Part model, mm, in its own coordinate system. Round coordinates to 2 decimals unless told otherwise and drop trailing zeros. Write each loop counter-clockwise with the first axis right and the second up, starting at its lowest first coordinate (ties: lowest second). Pieces come first, ordered by that corner, then holes. Notation, with made-up numbers: M 32,33 L 37,33 A19 cw 37,49 Z; hole C 11,37.5 d8. An arc over 180 degrees is marked long. Use a Markdown table: item, result. Add a question column.
1) Slice it at D-D on z = 4.75. Write the cut outline in (x, y) (1 decimal).
2) Slice it at C-C on z = 3.25. Write the cut outline in (x, y), plus the area to 3 significant figures.
3) Wall check: probe 1 along Y at (x, z) = (0, 1.5); probe 2 along Y at (x, z) = (0, 4.5); probe 3 along Y at (x, z) = (-7, 1.75). Give the ranges that are in metal, low to high.
4) Drop a flat-ended pin along its axis: P1, Ø1, axis at x = 5.5, z = 3, coming from the +Y side. Give the stop position or say it passes through.
5) Two-plate mould, pull along X, no slides. Class faces 1 (the face through (-2.17, -9.76, 1.97)), 2 (the face through (0, -2, 7)), 3 (the face through (6.2, -0.6, 3.5)): released by +X, released by -X, zero draft, split by the parting line, or undercut.
6) Slice it at A-A on y = 0. Write the cut outline in (x, z), plus the area to 4 significant figures.
```python
from build123d import *

# Parameters (mm, degrees)
SKETCH1_R           = 10
SKETCH1_R_2         = 1.6
BOSS_EXTRUDE1_DEPTH = 7
SKETCH2_R           = 1
CUT_EXTRUDE1_DEPTH  = 7
CHAMFER2_SIZE       = 3
CHAMFER2_SIZE2      = 1.25


with BuildPart() as part:
    # Sketch1 → Boss-Extrude1 (new body)
    with BuildSketch(Plane.XY):
        Circle(SKETCH1_R)
        Circle(SKETCH1_R_2, mode=Mode.SUBTRACT)
    extrude(amount=BOSS_EXTRUDE1_DEPTH)

    # Sketch2 → Cut-Extrude1 (cut)
    with BuildSketch(Plane.XY.offset(7)):
        with Locations((7, 0)):
            Circle(SKETCH2_R)
        with Locations((0, -7)):
            Circle(SKETCH2_R)
        with Locations((-7, 0)):
            Circle(SKETCH2_R)
        with Locations((0, 7)):
            Circle(SKETCH2_R)
    extrude(amount=-CUT_EXTRUDE1_DEPTH, mode=Mode.SUBTRACT)

    # Chamfer2
    chamfer2_edges = [part.edges().sort_by_distance(p)[0] for p in [
        (-10, 0, 7),
    ]]
    chamfer2_side = [part.faces().sort_by_distance(p)[0] for p in [
        (-10, 0, 3.5),
    ]]
    chamfer(chamfer2_edges, length=CHAMFER2_SIZE, length2=CHAMFER2_SIZE2, reference=chamfer2_side[0])


solid = part.part
```
Entries:
| question | item | result |
|---|---|---|
| 1 | outline | C 0,0 d19.4; hole C -7,0 d2; hole C 0,0 d3.2; hole C 0,-7 d2; hole C 0,7 d2; hole C 7,0 d2 |
| 2 | outline | C 0,0 d20; hole C -7,0 d2; hole C 0,0 d3.2; hole C 0,-7 d2; hole C 0,7 d2; hole C 7,0 d2 |
| 2 | area | 294 mm^2 |
| 3 | probe 1 | y = -10 to -8, -6 to -1.6, 1.6 to 6, 8 to 10 |
| 3 | probe 2 | y = -9.79 to -8, -6 to -1.6, 1.6 to 6, 8 to 9.79 |
| 3 | probe 3 | y = -7.14 to -1, 1 to 7.14 |
| 4 | P1 | stops at y = 8.66 |
| 5 | face 1 | split by the parting line |
| 5 | face 2 | zero draft |
| 5 | face 3 | undercut |
| 6 | outline | M -10,0 L -8,0 L -8,7 L -8.75,7 L -10,4 Z; M -6,0 L -1.6,0 L -1.6,7 L -6,7 Z; M 1.6,0 L 6,0 L 6,7 L 1.6,7 Z; M 8,0 L 10,0 L 10,4 L 8.75,7 L 8,7 Z |
| 6 | area | 85.85 mm^2 |
